Autodesk Inventor part; units mm, degrees
ref_plane "YZ Plane" through (0, 0, 0) normal (1, 0, 0) x (0, 1, 0)
ref_plane "XZ Plane" through (0, 0, 0) normal (0, 1, 0) x (-1, 0, 0)
ref_plane "XY Plane" through (0, 0, 0) normal (0, 0, 1) x (1, 0, 0)
sketch "Boceto1" plane through (0, 0, 0) normal (0, 0, 1) x (1, 0, 0)
  arc A0 (33.9935, 36.6667) -> (33.9935, -36.6667) centre (0, 0) ccw
  circle A1 centre (0, 0) radius 25
  line L0 (50.9902, 30) -> (180, 30)
  line L1 (180, 30) -> (180, -30)
  line L2 (180, -30) -> (50.9902, -30)
  arc A2 (33.9935, 36.6667) -> (50.9902, 30) centre (50.9902, 55) ccw
  arc A3 (50.9902, -30) -> (33.9935, -36.6667) centre (50.9902, -55) ccw
  dimension "d0" = 100
  dimension "d1" = 50
  dimension "d6" = 50
  dimension "d7" = 50
extrude "Extrusión1" add sketch "Boceto1" along normal blind 60
sketch "Boceto2" plane through (180, -30, 0) normal (1, 0, 0) x (0, 0, -1)
  line L0 (0, 60) -> (-60, 60)
  line L1 (0, 0) -> (0, 60)
  line L2 (0, 60) -> (-18.06, 60)
  line L3 (0, 60) -> (0, 41.94)
  line L4 (0, 80) -> (0, -20)
  line L5 (0, 41.94) -> (-18.06, 60)
  line L6 (-41.94, 60) -> (-60, 41.94)
  line L7 (-60, 60) -> (-60, 41.94)
  line L8 (-60, 60) -> (-41.94, 60)
  line L9 (-60, 18.06) -> (-41.94, 0)
  line L10 (-60, 0) -> (-41.94, 0)
  line L11 (-60, 0) -> (-60, 18.06)
  line L12 (-18.06, 0) -> (0, 18.06)
  line L13 (0, 0) -> (0, 18.06)
  line L14 (0, 0) -> (-18.06, 0)
  point P0 (0, 30)
  point P1 (-30, 30)
  point P2 (-30, 60)
  point P3 (0, 30)
  point P4 (0, 66.6667)
  point P5 (0, -6.6667)
  dimension "d11" = 18.06
  dimension "d12" = 18.06
  dimension "d15" = 360
extrude "Extrusión3" cut sketch "Boceto2" against normal blind 60
sketch "Boceto3" plane through (180, -11.94, 0) normal (1, 0, 0) x (0, 0, -1)
  circle A0 centre (-30, 11.94) radius 25
  line L0 (-18.06, 41.94) -> (-41.94, 41.94)
  line L1 (0, 0) -> (0, 23.88)
  point P0 (0, 11.94)
  point P1 (-30, 41.94)
  point P2 (0, 11.94)
  dimension "d21" = 50
extrude "Extrusión4" add sketch "Boceto3" along normal blind 120.5
fillet "Empalme1" radius 12 4 edges at (120, 20.97, 50.97) (120, 20.97, 9.03) (120, -20.97, 9.03) (120, -20.97, 50.97)
properties part number "Eye end" material "Stainless Steel, 440C"
Work out the finished part from the listing and answer in its coordinate system (mm). A direction names the side the tool comes from. Coordinates: 2 decimals unless noted, no trailing zeros. Loops run counter-clockwise (first coordinate to the right, second up) from the corner with the lowest first, then second, coordinate; pieces in that order, holes last.
1) Section D-D (x = 224.5) is taken. Give the vertices of the cut face in (y, z).
Results:
outline: circle Ø50 at (0, 30)
2) Section C-C (y = -3) is taken. Give the vertices of the cut face in (x, z), plus the area to 3 significant figures.
Results:
outline: (-49.91, 0) - (-24.82, 0) - (-24.82, 60) - (-49.91, 60) - close; (24.82, 0) - (180, 0) - (180, 5.18) - (300.5, 5.18) - (300.5, 54.82) - (180, 54.82) - (180, 60) - (24.82, 60) - close
area: 16,800 mm2
3) Flat-ended cylindrical pins translate along their axes: pin 1 (12 mm diameter, centred on y = -33, z = 7, fed in from -X); pin 2 (0.5 mm diameter, centred on y = -29.5, z = 59.5, fed in from +X); pin 3 (4 mm diameter, centred on x = 133, z = 27, fed in from +Y). Find the tip coordinate at first contact, or state that the pin passes through.
Results:
pin 1: stops at x = -42.08
pin 2: stops at x = 120
pin 3: stops at y = 30
4) For a pull along X with two mould halves and no side action, classify faces 1 (the cylindrical face through (23.846, -7.509, 29.58)), 2 (the cylindrical face through (41.98, 31.68, 29.58)), 3 (the cylindrical face through (-49.974, -1.623, 29.58)), 4 (the flat face through (156.34, -20.84, 51.1)) as +X half, -X half, draft (parallel to the pull), parting line (faces both ways), or undercut.
Results:
face 1: undercut
face 2: +X half
face 3: parting line
face 4: draft
5) For faces 5 (the flat face through (156.34, 20.84, 8.9)), 6 (the flat face through (180, 18, 48)), 7 (the flat face through (156.34, -21.1, 9.16)), determine the directions among +Z, -Z, +X, -X, +Y, -Y from which every point of the face is accessible in a straight line to the end or side of a thin tool.
Results:
face 5: -Z, +X, +Y
face 6: +X
face 7: -Z, +X, -Y
6) Consider probe 1 along Y at (x, z) = (0, 44); probe 2 along X at (y, z) = (-17.5, 31.5); probe 3 along Y at (x, z) = (80.5, 48). Determine where each line is inside the solid, lowest interval first.
Results:
probe 1: y = -50 to -25, 25 to 50
probe 2: x = -46.84 to -17.85, 17.85 to 300.5
probe 3: y = -30 to 30
7) Section B-B (z = 30) is taken. Give the vertices of the cut face in (x, y), plus the area to 3 significant figures.
Results:
outline: (33.99, -36.67) arc R25 cw to (50.99, -30) - (180, -30) - (180, -25) - (300.5, -25) - (300.5, 25) - (180, 25) - (180, 30) - (50.99, 30) arc R25 cw to (33.99, 36.67) arc R50 ccw (long way) to start; hole circle Ø50 at (0, 0)
area: 19,900 mm2
8) Section A-A (x = 0) is taken. Give the vertices of the cut face in (y, z), plus the area to 3 significant figures.
Results:
outline: (-50, 0) - (-25, 0) - (-25, 60) - (-50, 60) - close; (25, 0) - (50, 0) - (50, 60) - (25, 60) - close
area: 3,000 mm2
